from build123d import *

# Parameters (mm, degrees)
PAD_DEPTH          = 56
POLARPATTERN_COUNT = 6


with BuildPart() as part:
    # Sketch → Revolution002 (revolve)
    with BuildSketch(Plane.XZ):
        Polygon((19, 5.8085106383), (19, 75.5), (36.5, 75.5), (36.5, 73), (31, 73), (31, 22), (36.5, 22), (36.5, 19.5), (20, 5.8085106383), align=None)
    revolve(axis=Axis((0, 0, 0), (0, 0, 1)))

    # Sketch004 → Pad (new body)
    with BuildSketch(Plane.XY.offset(75.5)):
        with BuildLine():
            ThreePointArc((30.8991935484, -2.4979667851), (31, 0), (30.8991935484, 2.4979667851))
            ThreePointArc((30.8991935484, -2.4979667851), (33.5, 0), (30.8991935484, 2.4979667851))
        make_face()
    pad = extrude(amount=-PAD_DEPTH)

    # PolarPattern: Pad ×6 about axis
    polarpattern_axis = Axis((0, 0, 75.5), (0, 0, 1))
    for i in range(1, POLARPATTERN_COUNT):
        add(pad.rotate(polarpattern_axis, i * 360 / POLARPATTERN_COUNT))


solid = part.part
Model file for the job. Use its own axes, mm. A direction names the side the tool comes from. Give positions to 0.01 mm unless a question says otherwise; leave off trailing zeros. Loops run counter-clockwise (first coordinate to the right, second up) from the corner with the lowest first, then second, coordinate; pieces in that order, holes last. Notation, with made-up numbers: (-28.5, 74) -> (-9.5, 74) arc R24 ccw to (-9.5, 110) -> close; hole circle Ø8 at (40.25, 6). An arc over 180 degrees is marked (long way). Use a Markdown table: item, result. Add a question column.
(1) Slice it at B-B on z = 36. List the corners of the cut face in (x, y), and give its area (3 significant figures).
(2) Slice it at A-A on y = 0. List the corners of the cut face in (x, z), and give its area (3 significant figures).
(3) Tool access for faces 1 (the flat face through (-11, -30, 22)), 2 (the cylindrical face through (0, -31, 47)), 3 (the cylindrical face through (-7.912, -35.632, 20.732)): list every direction of +Z, -Z, +X, -X, +Y, -Y with a clear straight run to the whole face (end or side of a thin tool).
(4) Slice it at C-C on z = 13. List the corners of the cut face in (x, y), and give its area (3 significant figures).
(5) Drop flat-ended pins along their axis: pin 1 Ø12 at (y, z) = (6, 33) entering from +X; pin 2 Ø5 at (y, z) = (28, 35) entering from -X; pin 3 Ø2 at (x, z) = (12.5, 39) entering from +Y. Give the stop position or say it passes through.
(6) Wall check: line 1 along Z through (x, y) = (23.5, 26); line 2 along Y through (x, z) = (-28, 57); line 3 along Y through (x, z) = (15.5, 65). Give the ranges that are in metal, low to high.
(7) Mould opens along Y. For faces 4 (the cylindrical face through (0, 31, 47)), 5 (the cylindrical face through (33.5, -0.1, 47.9)), 6 (the cylindrical face through (-16.8, -28.98, 47.86)), 7 (the cylindrical face through (16.8, 28.98, 47.86)) say: +Y half, -Y half, draft (parallel to the pull), parting line (faces both ways), or undercut.
Filled sheet:
| question | item | result |
|---|---|---|
| 1 | outline | (-30.9, -2.5) arc R31 ccw to (-17.61, -25.51) arc R2.5 ccw (long way) to (-13.29, -28.01) arc R31 ccw to (13.29, -28.01) arc R2.5 ccw (long way) to (17.61, -25.51) arc R31 ccw to (30.9, -2.5) arc R2.5 ccw (long way) to (30.9, 2.5) arc R31 ccw to (17.61, 25.51) arc R2.5 ccw (long way) to (13.29, 28.01) arc R31 ccw to (-13.29, 28.01) arc R2.5 ccw (long way) to (-17.61, 25.51) arc R31 ccw to (-30.9, 2.5) arc R2.5 ccw (long way) to start; hole circle Ø38 at (0, 0) |
| 1 | area | 1,940 mm2 |
| 2 | outline | (-36.5, 19.5) -> (-20, 5.81) -> (-19, 5.81) -> (-19, 75.5) -> (-36.5, 75.5) -> (-36.5, 73) -> (-33.5, 73) -> (-33.5, 22) -> (-36.5, 22) -> close; (19, 5.81) -> (20, 5.81) -> (36.5, 19.5) -> (36.5, 22) -> (33.5, 22) -> (33.5, 73) -> (36.5, 73) -> (36.5, 75.5) -> (19, 75.5) -> close |
| 2 | area | 1,910 mm2 |
| 3 | face 1 | none |
| 3 | face 2 | -Y |
| 3 | face 3 | +Z, -Z |
| 4 | outline | circle Ø57.33 at (0, 0); hole circle Ø38 at (0, 0) |
| 4 | area | 1,450 mm2 |
| 5 | pin 1 | x = 33.5 |
| 5 | pin 2 | x = -18 |
| 5 | pin 3 | y = 28.79 |
| 6 | line 1 | 18.29 to 22, 73 to 75.5 |
| 6 | line 2 | -13.3 to 13.3 |
| 6 | line 3 | -29.35 to -10.99, 10.99 to 29.35 |
| 7 | face 4 | +Y half |
| 7 | face 5 | parting line |
| 7 | face 6 | undercut |
| 7 | face 7 | undercut |
